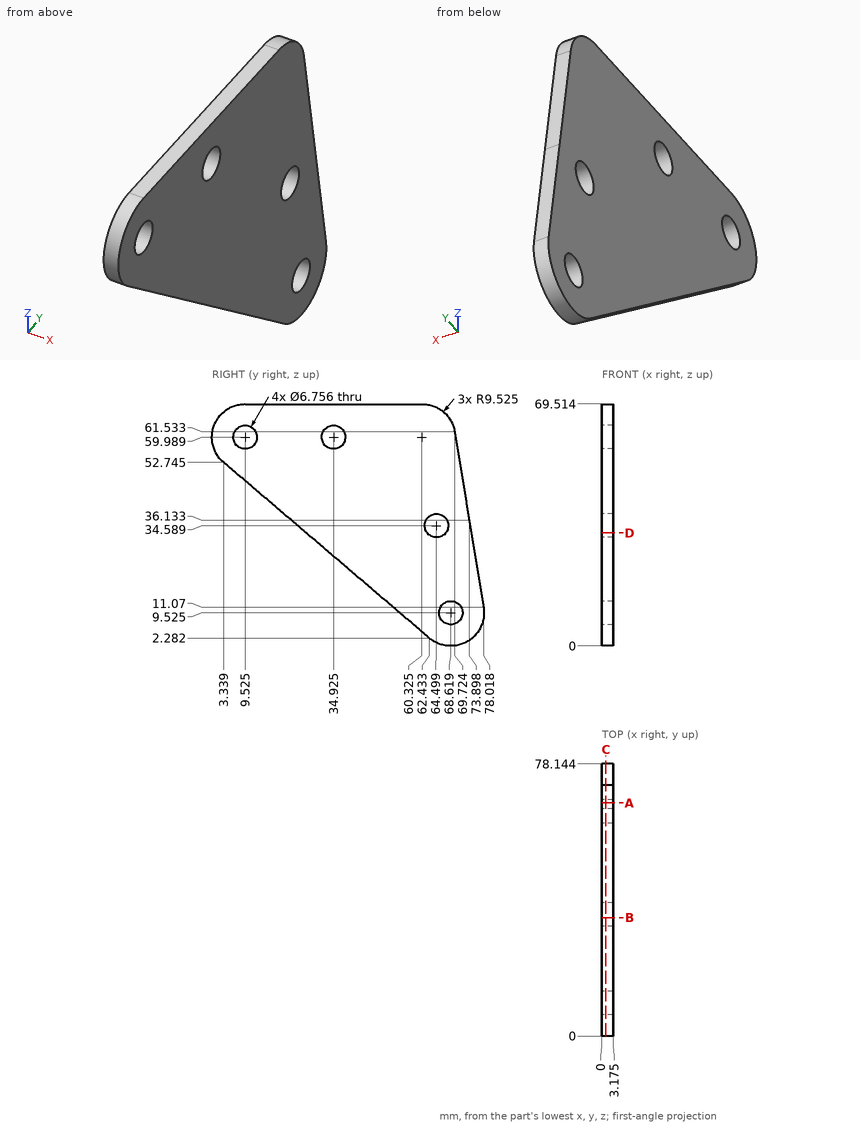
Answer from the drawing. Dimensions are ordinates in mm from the lowest x, y and z of the part. Round coordinates to 2 decimals unless told otherwise and drop trailing zeros. Write each loop counter-clockwise with the first axis right and the second up, starting at its lowest first coordinate (ties: lowest second). Pieces come first, ordered by that corner, then holes. Notation, with made-up numbers: (5, 31.5) - (46, 31.5) arc R21 cw to (46, 48.5) - close; hole circle Ø1 at (64, 46.5). An arc over 180 degrees is marked (long way). One line per item, written item: value.
Q1. Find section A-A (y = 67). Determine the outline of the cut face in (x, z) (1 decimal), and give its area (3 significant figures).
The answers:
outline: (0, 0.1) - (3.2, 0.1) - (3.2, 6.6) - (0, 6.6) - close; (0, 12.5) - (3.2, 12.5) - (3.2, 32.3) - (0, 32.3) - close; (0, 36.9) - (3.2, 36.9) - (3.2, 66.8) - (0, 66.8) - close
area: 178 mm2
Q2. Find section C-C (x = 1.15). Count the separate pieces of the cut face and the enclosed holes in it, and give its area (3 significant figures).
The answers:
separate pieces: 1
enclosed holes: 4
area: 3,130 mm2
Q3. Straight lines are drawn through the part: line 1 (Y direction, x = 0.2, z = 60) (1 decimal); line 2 (Y direction, x = 2.25, z = 57.5) (1 decimal); line 3 (Z direction, x = 2.45, y = 35.5) (1 decimal). For each, find the intervals that lie inside material, in ascending order. Write a range as from..to.
The answers:
line 1: y = 0..6.1, 12.9..31.5, 38.3..70
line 2: y = 0.3..7.2, 11.8..32.6, 37.2..70.4
line 3: z = 25.3..56.7, 63.3..69.5
Q4. Find section D-D (z = 32.5). Determine the outline of the cut face in (x, y) (1 decimal), and give its area (3 significant figures).
The answers:
outline: (0, 27) - (3.2, 27) - (3.2, 61.8) - (0, 61.8) - close; (0, 67.2) - (3.2, 67.2) - (3.2, 74.5) - (0, 74.5) - close
area: 134 mm2
Q5. Each of these flat-tipped pins is pushed along its axis until it touches: P1, Ø12, axis at y = 8.5, z = 51, coming from the -X side; P2, Ø1, axis at x = 1, z = 23.5, coming from the -Y side; P3, Ø6, axis at y = 34.92, z = 59.99, coming from the -X side. Where does it stop, or does it pass through?
The answers:
P1: stops at x = 0
P2: stops at y = 37
P3: passes through
Q6. Find section B-B (y = 34). Determine the outline of the cut face in (x, z) (1 decimal), and give its area (3 significant figures).
The answers:
outline: (0, 26.6) - (3.2, 26.6) - (3.2, 56.7) - (0, 56.7) - close; (0, 63.2) - (3.2, 63.2) - (3.2, 69.5) - (0, 69.5) - close
area: 116 mm2
